```python
from build123d import *

# Parameters (mm, degrees)
SKETCH1_W                = 94
SKETCH1_H                = 69
PI_BASE_DEPTH            = 3
SKETCH2_W                = 94
SKETCH2_H                = 69
SKETCH2_W_2              = 86
SKETCH2_H_2              = 57
PI_WALLS_DEPTH           = 29
SKETCH4_R                = 2.5
STAND_OFFS_DEPTH         = 3
SKETCH6_R                = 1.5
PI_MOUNT_HOLES_DEPTH     = 6
STANDOFF_FILLET_R        = 2
SKETCH5_W                = 54
SKETCH5_H                = 29
HDMI_AUX_CUT_DEPTH       = 3
SKETCH10_W               = 15
SKETCH10_H               = 29
PWR_CUT_THROUGH_DEPTH    = 3
SKETCH3_W                = 16.6
SKETCH3_H                = 24.6
SKETCH3_W_2              = 13.6
SKETCH3_H_2              = 23
ETH_USB_CUT_DEPTH        = 3
SKETCH8_W                = 1
SKETCH8_H                = 15.6
USB_FLANGE_CUT_DEPTH     = 24
SKETCH16_W               = 15
SKETCH16_H               = 27
SD_CUT_DEPTH             = 3
SKETCH12_R               = 1.4
PCA_MOUNTING_CUT_DEPTH   = 4.4
SKETCH13_R               = 6
CAP_WIRE_HOLE_DEPTH      = 5
SKETCH15_W               = 76
SKETCH15_H               = 24
SIDE_PANEL_CUT_DEPTH     = 6
USB_TOP_TRIM_REACH       = 107.12
SKETCH17_W               = 37.6
SKETCH17_H               = 8
SKETCH18_R               = 1.4
TOP_MOUNTING_HOLES_DEPTH = 5
PCA_POWER_CUT_REACH      = 105.336
SKETCH19_W               = 15
SKETCH19_H               = 10


with BuildPart() as part:
    # Sketch1 → pi_base (new body)
    with BuildSketch(Plane(origin=(0, 0, 0), x_dir=(1, 0, 0), z_dir=(0, 1, 0))):
        Rectangle(SKETCH1_W, SKETCH1_H)
    extrude(amount=PI_BASE_DEPTH)

    # Sketch2 → pi_walls (add)
    with BuildSketch(Plane(origin=(0, 3, 0), x_dir=(1, 0, 0), z_dir=(0, 1, 0))):
        Rectangle(SKETCH2_W, SKETCH2_H)
        with Locations((-1, 0)):
            Rectangle(SKETCH2_W_2, SKETCH2_H_2, mode=Mode.SUBTRACT)
    extrude(amount=PI_WALLS_DEPTH)

    # Sketch4 → stand_offs (add)
    with BuildSketch(Plane(origin=(0, 3, 0), x_dir=(1, 0, 0), z_dir=(0, 1, 0))):
        with Locations(Location((-19.6, 24.5, 0), (0, 0, 270))):
            Circle(SKETCH4_R)
        with Locations(Location((38.4, 24.5, 0), (0, 0, 270))):
            Circle(SKETCH4_R)
        with Locations(Location((-19.6, -24.5, 0), (0, 0, 270))):
            Circle(SKETCH4_R)
        with Locations(Location((38.4, -24.5, 0), (0, 0, 270))):
            Circle(SKETCH4_R)
    extrude(amount=STAND_OFFS_DEPTH)

    # Sketch6 → pi_mount_holes (cut)
    with BuildSketch(Plane(origin=(0, 6, 0), x_dir=(1, 0, 0), z_dir=(0, 1, 0))):
        with Locations(Location((-19.6, 24.5, 0), (0, 0, 270))):
            Circle(SKETCH6_R)
        with Locations(Location((38.4, 24.5, 0), (0, 0, 270))):
            Circle(SKETCH6_R)
        with Locations(Location((-19.6, -24.5, 0), (0, 0, 270))):
            Circle(SKETCH6_R)
        with Locations(Location((38.4, -24.5, 0), (0, 0, 270))):
            Circle(SKETCH6_R)
    extrude(amount=-PI_MOUNT_HOLES_DEPTH, mode=Mode.SUBTRACT)

    # standoff_fillet
    # the kernel refuses this fillet: 2 mm, written as the material it adds along each edge
    with BuildSketch(Plane(origin=(-19.6, 3, -24.5), x_dir=(0, 0, 1), z_dir=(-1, 0, 0))) as standoff_fillet_piece_1:
        with BuildLine():
            CenterArc((2.5 + STANDOFF_FILLET_R, STANDOFF_FILLET_R), STANDOFF_FILLET_R, 180, 90)
            Line((2.5, STANDOFF_FILLET_R), (2.5, 0))
            Line((2.5, 0), (2.5 + STANDOFF_FILLET_R, 0))
        make_face()
    revolve(axis=Axis((-19.6, 3, -24.5), (0, 1, 0)))
    with BuildSketch(Plane(origin=(38.4, 3, -24.5), x_dir=(0, 0, 1), z_dir=(-1, 0, 0))) as standoff_fillet_piece_2:
        with BuildLine():
            CenterArc((2.5 + STANDOFF_FILLET_R, STANDOFF_FILLET_R), STANDOFF_FILLET_R, 180, 90)
            Line((2.5, STANDOFF_FILLET_R), (2.5, 0))
            Line((2.5, 0), (2.5 + STANDOFF_FILLET_R, 0))
        make_face()
    revolve(axis=Axis((38.4, 3, -24.5), (0, 1, 0)))
    with BuildSketch(Plane(origin=(38.4, 3, 24.5), x_dir=(0, 0, 1), z_dir=(-1, 0, 0))) as standoff_fillet_piece_3:
        with BuildLine():
            CenterArc((2.5 + STANDOFF_FILLET_R, STANDOFF_FILLET_R), STANDOFF_FILLET_R, 180, 90)
            Line((2.5, STANDOFF_FILLET_R), (2.5, 0))
            Line((2.5, 0), (2.5 + STANDOFF_FILLET_R, 0))
        make_face()
    revolve(axis=Axis((38.4, 3, 24.5), (0, 1, 0)))
    with BuildSketch(Plane(origin=(-19.6, 3, 24.5), x_dir=(0, 0, 1), z_dir=(-1, 0, 0))) as standoff_fillet_piece_4:
        with BuildLine():
            CenterArc((2.5 + STANDOFF_FILLET_R, STANDOFF_FILLET_R), STANDOFF_FILLET_R, 180, 90)
            Line((2.5, STANDOFF_FILLET_R), (2.5, 0))
            Line((2.5, 0), (2.5 + STANDOFF_FILLET_R, 0))
        make_face()
    revolve(axis=Axis((-19.6, 3, 24.5), (0, 1, 0)))

    # Sketch5 → hdmi_aux_cut (cut)
    with BuildSketch(Plane.XY.offset(-28.5)):
        with Locations((12, 17.5)):
            Rectangle(SKETCH5_W, SKETCH5_H)
    extrude(amount=-HDMI_AUX_CUT_DEPTH, mode=Mode.SUBTRACT)

    # Sketch10 → pwr_cut_through (cut)
    with BuildSketch(Plane.XY.offset(-31.5)):
        with Locations((31.5, 17.5)):
            Rectangle(SKETCH10_W, SKETCH10_H)
    extrude(amount=-PWR_CUT_THROUGH_DEPTH, mode=Mode.SUBTRACT)

    # Sketch3 → eth_usb_cut (cut)
    with BuildSketch(Plane.ZY.offset(47)):
        with Locations((-17.8, 19.7)):
            Rectangle(SKETCH3_W, SKETCH3_H)
        with Locations((1.1, 20.5)):
            Rectangle(SKETCH3_W_2, SKETCH3_H_2)
        with Locations((19.3, 20.5)):
            Rectangle(SKETCH3_W_2, SKETCH3_H_2)
    extrude(amount=-ETH_USB_CUT_DEPTH, mode=Mode.SUBTRACT)

    # Sketch8 → usb_flange_cut (cut)
    with BuildSketch(Plane(origin=(0, 32, 0), x_dir=(1, 0, 0), z_dir=(0, 1, 0))):
        with Locations((-45.5, -1.1)):
            Rectangle(SKETCH8_W, SKETCH8_H)
        with Locations((-45.5, -19.3)):
            Rectangle(SKETCH8_W, SKETCH8_H)
    extrude(amount=-USB_FLANGE_CUT_DEPTH, mode=Mode.SUBTRACT)

    # Sketch16 → sd_cut (cut)
    with BuildSketch(Plane.ZY.offset(-42)):
        with Locations((0, 18.5)):
            Rectangle(SKETCH16_W, SKETCH16_H)
    extrude(amount=-SD_CUT_DEPTH, mode=Mode.SUBTRACT)

    # Sketch12 → pca_mounting_cut (cut)
    with BuildSketch(Plane(origin=(47, 0, 0), x_dir=(0, 0, -1), z_dir=(1, 0, 0))):
        with Locations((-28, 25.5)):
            Circle(SKETCH12_R)
        with Locations((-28, 6.5)):
            Circle(SKETCH12_R)
        with Locations((28, 6.5)):
            Circle(SKETCH12_R)
        with Locations((28, 25.5)):
            Circle(SKETCH12_R)
    extrude(amount=-PCA_MOUNTING_CUT_DEPTH, mode=Mode.SUBTRACT)

    # Sketch13 → cap_wire_hole (cut)
    with BuildSketch(Plane.ZY.offset(-42)):
        with Locations((19.5, 24)):
            Circle(SKETCH13_R)
    extrude(amount=-CAP_WIRE_HOLE_DEPTH, mode=Mode.SUBTRACT)

    # Sketch15 → side_panel_cut (cut)
    with BuildSketch(Plane.XY.offset(34.5)):
        with Locations((0, 20)):
            Rectangle(SKETCH15_W, SKETCH15_H)
    extrude(amount=-SIDE_PANEL_CUT_DEPTH, mode=Mode.SUBTRACT)

    # usb_top_trim: up to this face of the body (flat: up to its plane)
    usb_top_trim_end = Plane(part.part.faces().sort_by_distance((-38, 20, 31.5))[0])
    # Sketch17 → usb_top_trim (cut, up to the picked face)
    with BuildSketch(Plane.ZY.offset(47), mode=Mode.PRIVATE) as usb_top_trim_sk1:
        with Locations((9.3, 28)):
            Rectangle(SKETCH17_W, SKETCH17_H)
    usb_top_trim_tool1 = split(extrude(usb_top_trim_sk1.sketch, amount=-USB_TOP_TRIM_REACH, mode=Mode.PRIVATE), bisect_by=usb_top_trim_end, keep=Keep.BOTH, mode=Mode.PRIVATE)
    add(usb_top_trim_tool1.solids().sort_by(Axis((-47, 28, 9.3), (1, 0, 0)))[0], mode=Mode.SUBTRACT)

    # Sketch18 → top_mounting_holes (cut)
    with BuildSketch(Plane(origin=(0, 32, 0), x_dir=(1, 0, 0), z_dir=(0, 1, 0))):
        with Locations(Location((-44, 31.2, 0), (0, 0, 270))):
            Circle(SKETCH18_R)
        with Locations(Location((44, 31.2, 0), (0, 0, 270))):
            Circle(SKETCH18_R)
        with Locations(Location((44, -31.2, 0), (0, 0, 270))):
            Circle(SKETCH18_R)
        with Locations(Location((-44, -31.2, 0), (0, 0, 270))):
            Circle(SKETCH18_R)
    extrude(amount=-TOP_MOUNTING_HOLES_DEPTH, mode=Mode.SUBTRACT)

    # Sketch19 → pca_power_cut (cut, up to next)
    with BuildSketch(Plane.ZY.offset(-45), mode=Mode.PRIVATE) as pca_power_cut_sk1:
        with Locations((0, 27)):
            Rectangle(SKETCH19_W, SKETCH19_H)
    pca_power_cut_tool1 = extrude(pca_power_cut_sk1.sketch, amount=-PCA_POWER_CUT_REACH, mode=Mode.PRIVATE) & part.part
    add(pca_power_cut_tool1.solids().sort_by_distance((45, 27, 0))[0], mode=Mode.SUBTRACT)


solid = part.part
```
Part model, mm, in its own coordinate system. A direction names the side the tool comes from. Round coordinates to 2 decimals unless told otherwise and drop trailing zeros. Order: outer loops, then holes, each group sorted by start corner. A loop starts at its lowest first (then second) coordinate and runs counter-clockwise, first axis right, second up. Notation, with made-up numbers: M 87.25,88.25 L 135.25,88.25 A18 ccw 135.25,104.25 Z; hole C 13.25,69.25 d3. An arc over 180 degrees is marked long. Put each result on its own line as item: value. Start each with the question number.
1. Slice it at A-A on x = -19.6. List the corners of the cut face in (y, z).
2. Tool access for faces 1 (the face through (-46, 8.3, 2.3)), 2 (the face through (24, 17, -33)), 3 (the face through (-46, 24, 10)), 4 (the face through (44.831, 24.133, 28.303)), 5 (the face through (-38, 20, 32)): list every direction of +Z, -Z, +X, -X, +Y, -Y with a clear straight run to the whole face (end or side of a thin tool).
3. Slice it at B-B on x = 44. List the corners of the cut face in (y, z), then the cut area to 3 significant figures.
4. Two-plate mould, pull along X, no slides. Class faces 6 (the face through (42.6, 7, -28)), 7 (the face through (44.83, 6.56, 29.4)), 8 (the face through (44, 21, -7.5)), 9 (the face through (37, 6, -23)): +X half, -X half, draft (parallel to the pull), parting line (faces both ways), or undercut.
5. Drop flat-ended pins along their axis: pin 1 (3.5 mm diameter, centred on x = -44, z = 31.2, fed in from -Y); pin 2 (2.5 mm diameter, centred on x = 44, z = 31.2, fed in from +Y); pin 3 (6 mm diameter, centred on x = 25, y = 22, fed in from +Z); pin 4 (0.5 mm diameter, centred on x = -44.5, z = 17, fed in from +Y). Give the stop position or say it passes through.
6. Drill centre lines: probe 1 along Y at (x, z) = (45.45, 28); probe 2 along Z at (x, y) = (-31, 5); probe 3 along Z at (x, y) = (21, 6.5). Where is each one in solid material? Low to high. Write a range as [from, to].
7. Slice it at D-D on z = -24.5. List the corners of the cut face in (x, y), then the cut area to 3 significant figures.
8. Slice it at C-C on y = 15. State how many separate pieces and enclosed holes the cut face has, then the cut area to 3 significant figures.
Findings:
1. outline: M 0,-34.5 L 32,-34.5 L 32,-28.5 L 3.06,-28.5 A2 cw 5,-27 L 6,-27 L 6,-26 L 0,-26 Z; M 0,-23 L 6,-23 L 6,-22 L 5,-22 A2 cw 3,-20 L 3,20 A2 cw 5,22 L 6,22 L 6,23 L 0,23 Z; M 0,26 L 6,26 L 6,27 L 5,27 A2 cw 3.06,28.5 L 8,28.5 L 8,34.5 L 0,34.5 Z
2. face 1: +Y
2. face 2: -Z, +Y
2. face 3: -X, +Y
2. face 4: +X
2. face 5: +Z, +Y
3. outline: M 0,-34.5 L 32,-34.5 L 32,-32.6 L 27,-32.6 L 27,-29.8 L 32,-29.8 L 32,-7.5 L 5,-7.5 L 5,7.5 L 32,7.5 L 32,29.8 L 27,29.8 L 27,32.6 L 32,32.6 L 32,34.5 L 0,34.5 Z; hole C 6.5,-28 d2.8; hole C 6.5,28 d2.8; hole C 24,19.5 d12; hole C 25.5,-28 d2.8; hole C 25.5,28 d2.8
3. area: 1,640 mm2
4. face 6: +X half
4. face 7: draft
4. face 8: undercut
4. face 9: undercut
5. pin 1: y = 0
5. pin 2: y = 27
5. pin 3: z = -31.5
5. pin 4: y = 9
6. probe 1: [0, 5.1], [7.9, 24.1], [26.9, 32]
6. probe 2: [-34.5, -28.5], [28.5, 34.5]
6. probe 3: [-34.5, -31.5], [28.5, 34.5]
7. outline: M -47,0 L -21.1,0 L -21.1,6 L -22.1,6 L -22.1,5 A2 cw -24.1,3 L -44,3 L -44,7.4 L -47,7.4 Z; M -18.1,0 L 36.9,0 L 36.9,6 L 35.9,6 L 35.9,5 A2 cw 33.9,3 L -15.1,3 A2 cw -17.1,5 L -17.1,6 L -18.1,6 Z; M 39.9,0 L 47,0 L 47,32 L 42,32 L 42,3.21 A2 cw 40.9,5 L 40.9,6 L 39.9,6 Z
7. area: 438 mm2
8. separate pieces: 5
8. enclosed holes: 0
8. area: 741 mm2
